Design review of the part built by this model. Coordinates are the model's own, in mm. Face numbers are marked on the shaded views. A direction names the side the tool comes from. Round coordinates to 2 decimals unless told otherwise and drop trailing zeros. Order: outer loops, then holes, each group sorted by start corner. A loop starts at its lowest first (then second) coordinate and runs counter-clockwise, first axis right, second up. Notation, with made-up numbers: M 84.5,12.25 L 123.5,12.25 A11 cw 123.5,26.25 Z; hole C 42,47 d3. An arc over 180 degrees is marked long. Write each question's results on one line, items separated by ' | '. Start each with the question number.
Item 1: Wall thickness on line 1 (Z direction, x = 20, y = 0.9); line 2 (X direction, y = -0.45, z = -0.5); line 3 (X direction, y = -1.5, z = -0.5): over which ranges is each line inside the solid? List them lowest first. Write a range as [from, to].
Item 2: Clearance check with flat-ended pins moving along their axes: pin 1 (2 mm diameter, centred on y = -1, z = -3.5, fed in from +X); pin 2 (3 mm diameter, centred on x = 20, z = 0, fed in from -Y); pin 3 (0.8 mm diameter, centred on y = -1.5, z = -1, fed in from -X); pin 4 (1 mm diameter, centred on y = 0, z = 1, fed in from +X). State where each tip first meets the part, or that it passes through.
Item 3: Take a section at B-B, the plane z = 0. Write out the cut boundary in (x, y).
Item 4: Take a section at C-C, the plane x = 40. Write out the cut boundary in (y, z), plus the area to 3 significant figures.
Item 5: Machinability: for the marked faces 1 and 2, which of the approach directions +Z, -Z, +X, -X, +Y, -Y give a long, thin tool a straight path to every point of the face, cutting with its end or side? Answer none if there is none.
Item 6: Take a section at A-A, the plane x = 1. Write out the cut boundary in (y, z).
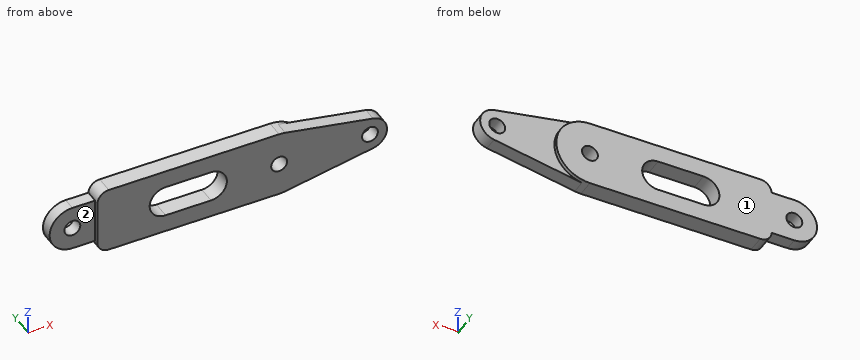
Autodesk Inventor part; units mm, degrees
ref_plane "YZ Plane" through (0, 0, 0) normal (1, 0, 0) x (0, 1, 0)
ref_plane "XZ Plane" through (0, 0, 0) normal (0, 1, 0) x (-1, 0, 0)
ref_plane "XY Plane" through (0, 0, 0) normal (0, 0, 1) x (1, 0, 0)
sketch "Sketch1" plane through (0, 0, 0) normal (0, 1, 0) x (-1, 0, 0)
  line L0 (-5, 0) -> (5, 0) construction
  line L1 (-5, -3.5) -> (5, -3.5)
  line L2 (5, 3.5) -> (-5, 3.5)
  arc A0 (-5, 3.5) -> (-5, -3.5) centre (-5, 0) ccw
  arc A1 (5, -3.5) -> (5, 3.5) centre (5, 0) ccw
  circle A2 centre (-20, 0) radius 1.75
  arc A3 (-20, 7.4) -> (-20, -7.4) centre (-20, 0) ccw
  line L3 (17.5, -7.4) -> (-20, -7.4)
  line L4 (17.5, 7.4) -> (-20, 7.4)
  line L5 (20, 4.9) -> (20, -4.9)
  arc A4 (25, -5) -> (25, 5) centre (25, 0) ccw
  circle A5 centre (25, 0) radius 1.75
  line L6 (25, 5) -> (19.998, 5)
  line L7 (25, -5) -> (19.998, -5)
  arc A6 (20, 4.9) -> (17.5, 7.4) centre (17.5, 4.9) ccw
  arc A7 (17.5, -7.4) -> (20, -4.9) centre (17.5, -4.9) ccw
  circle A8 centre (-40, 0) radius 1.75
  circle A9 centre (-40, 0) radius 3.75
  line L8 (-40, 3.75) -> (-21.3747, 7.2712)
  line L9 (-40, -3.75) -> (-21.3747, -7.2712)
  point P0 (0, 0)
  dimension "d3" = 10
  dimension "d4" = 3.5
  dimension "d5" = 3.5
  dimension "d6" = 14.8
  dimension "d10" = 10
  dimension "d11" = 5
  dimension "d12" = 3.5
  dimension "d13" = 2.5
  dimension "d51" = 15
  dimension "d52" = 40
  dimension "d53" = 3.5
  dimension "d54" = 7.5
  dimension "d55" = 20
extrude "Extrusion1" add sketch "Sketch1" along normal mid plane 3.8 contours L4 A6 L5 A7 L3 A3
sketch "Sketch4" plane through (0, 0, 0) normal (0, 1, 0) x (-1, 0, 0)
  line L0 (-5, 0) -> (5, 0) construction
  line L1 (-5, -3.5) -> (5, -3.5)
  line L2 (5, 3.5) -> (-5, 3.5)
  arc A0 (-5, 3.5) -> (-5, -3.5) centre (-5, 0) ccw
  arc A1 (5, -3.5) -> (5, 3.5) centre (5, 0) ccw
  circle A2 centre (-20, 0) radius 1.75
  arc A3 (-20, 7.4) -> (-20, -7.4) centre (-20, 0) ccw
  line L3 (17.5, -7.4) -> (-20, -7.4)
  line L4 (17.5, 7.4) -> (-20, 7.4)
  line L5 (20, 4.9) -> (20, -4.9)
  arc A4 (25, -5) -> (25, 5) centre (25, 0) ccw
  circle A5 centre (25, 0) radius 1.75
  line L6 (25, 5) -> (19.998, 5)
  line L7 (25, -5) -> (19.998, -5)
  arc A6 (20, 4.9) -> (17.5, 7.4) centre (17.5, 4.9) ccw
  arc A7 (17.5, -7.4) -> (20, -4.9) centre (17.5, -4.9) ccw
  circle A8 centre (-40, 0) radius 1.75
  arc A9 (-40.6844, 3.687) -> (-40.6844, -3.687) centre (-40, 0) ccw
  line L8 (-21.3505, 7.2757) -> (-40.6844, 3.687)
  arc A10 (-20, 7.4) -> (-20, -7.4) centre (-20, 0) ccw
  line L9 (-48.2908, 0) -> (-20.7624, 0) construction
  line L10 (-40.6844, -3.687) -> (-21.3505, -7.2757)
  point P0 (0, 0)
  point P1 (0, 0)
  dimension "d56" = 10
  dimension "d57" = 3.5
  dimension "d58" = 3.5
  dimension "d59" = 14.8
  dimension "d60" = 10
  dimension "d61" = 5
  dimension "d62" = 3.5
  dimension "d63" = 2.5
  dimension "d64" = 15
  dimension "d65" = 40
  dimension "d66" = 3.5
  dimension "d67" = 7.5
  dimension "d68" = 20
extrude "Extrusion4" add sketch "Sketch4" along normal blind 1.1 and the other way blind 1.9 contours A3 L10 A9 L8
sketch "Sketch5" plane through (0, 0, 0) normal (0, 1, 0) x (-1, 0, 0)
  line L0 (-5, 0) -> (5, 0) construction
  line L1 (-5, -3.5) -> (5, -3.5)
  line L2 (5, 3.5) -> (-5, 3.5)
  arc A0 (-5, 3.5) -> (-5, -3.5) centre (-5, 0) ccw
  arc A1 (5, -3.5) -> (5, 3.5) centre (5, 0) ccw
  circle A2 centre (-20, 0) radius 1.75
  arc A3 (-20, 7.4) -> (-20, -7.4) centre (-20, 0) ccw
  line L3 (17.5, -7.4) -> (-20, -7.4)
  line L4 (17.5, 7.4) -> (-20, 7.4)
  line L5 (20, 4.9) -> (20, -4.9)
  arc A4 (25, -5) -> (25, 5) centre (25, 0) ccw
  circle A5 centre (25, 0) radius 1.75
  line L6 (25, 5) -> (19.998, 5)
  line L7 (25, -5) -> (19.998, -5)
  arc A6 (20, 4.9) -> (17.5, 7.4) centre (17.5, 4.9) ccw
  arc A7 (17.5, -7.4) -> (20, -4.9) centre (17.5, -4.9) ccw
  circle A8 centre (-40, 0) radius 1.75
  circle A9 centre (-40, 0) radius 3.75
  line L8 (-40, 3.75) -> (-21.3747, 7.2712)
  line L9 (-40, -3.75) -> (-21.3747, -7.2712)
  point P0 (0, 0)
  point P1 (0, 0)
  dimension "d73" = 10
  dimension "d74" = 3.5
  dimension "d75" = 3.5
  dimension "d76" = 14.8
  dimension "d77" = 10
  dimension "d78" = 5
  dimension "d79" = 3.5
  dimension "d80" = 2.5
  dimension "d81" = 15
  dimension "d82" = 40
  dimension "d83" = 3.5
  dimension "d84" = 7.5
  dimension "d85" = 20
extrude "Extrusion5" add sketch "Sketch5" along normal blind 1.9 and the other way blind 0.8 contours L6 A4 L7 A7 L5 A6
move faces "Move1" translate (0, -0.1, 0) faces at (-21.0833, -0.8, 0)
Results list:
1) line 1: [-7.4, -1.75], [1.75, 7.4] | line 2: [-29.97, -26.68], [-23.32, -8.46], [8.46, 18.32], [21.68, 38.32], [41.68, 43.72] | line 3: [-20, -8.46], [8.46, 18.32], [21.68, 38.32], [41.68, 43.72]
2) pin 1: x = 42.8 | pin 2: through | pin 3: x = -20 | pin 4: x = 43.72
3) outline: M -30,-0.9 L -26.75,-0.9 L -26.75,1.9 L -30,1.9 Z; M -23.25,-0.9 L -20,-0.9 L -20,-1.9 L -8.5,-1.9 L -8.5,1.9 L -23.25,1.9 Z; M 8.5,-1.9 L 18.25,-1.9 L 18.25,1.9 L 8.5,1.9 Z; M 21.75,-1.9 L 38.25,-1.9 L 38.25,1.1 L 27.4,1.1 L 27.4,1.9 L 21.75,1.9 Z; M 41.75,-1.9 L 43.75,-1.9 L 43.75,1.1 L 41.75,1.1 Z
4) outline: M -1.9,-3.81 L 1.1,-3.81 L 1.1,-1.75 L -1.9,-1.75 Z; M -1.9,1.75 L 1.1,1.75 L 1.1,3.81 L -1.9,3.81 Z | area: 12.4 mm²
5) face 1: +Z, -Z, +X, -X, +Y | face 2: +Z, -Z, -X, -Y
6) outline: M -1.9,-7.4 L 1.9,-7.4 L 1.9,-3.5 L -1.9,-3.5 Z; M -1.9,3.5 L 1.9,3.5 L 1.9,7.4 L -1.9,7.4 Z
